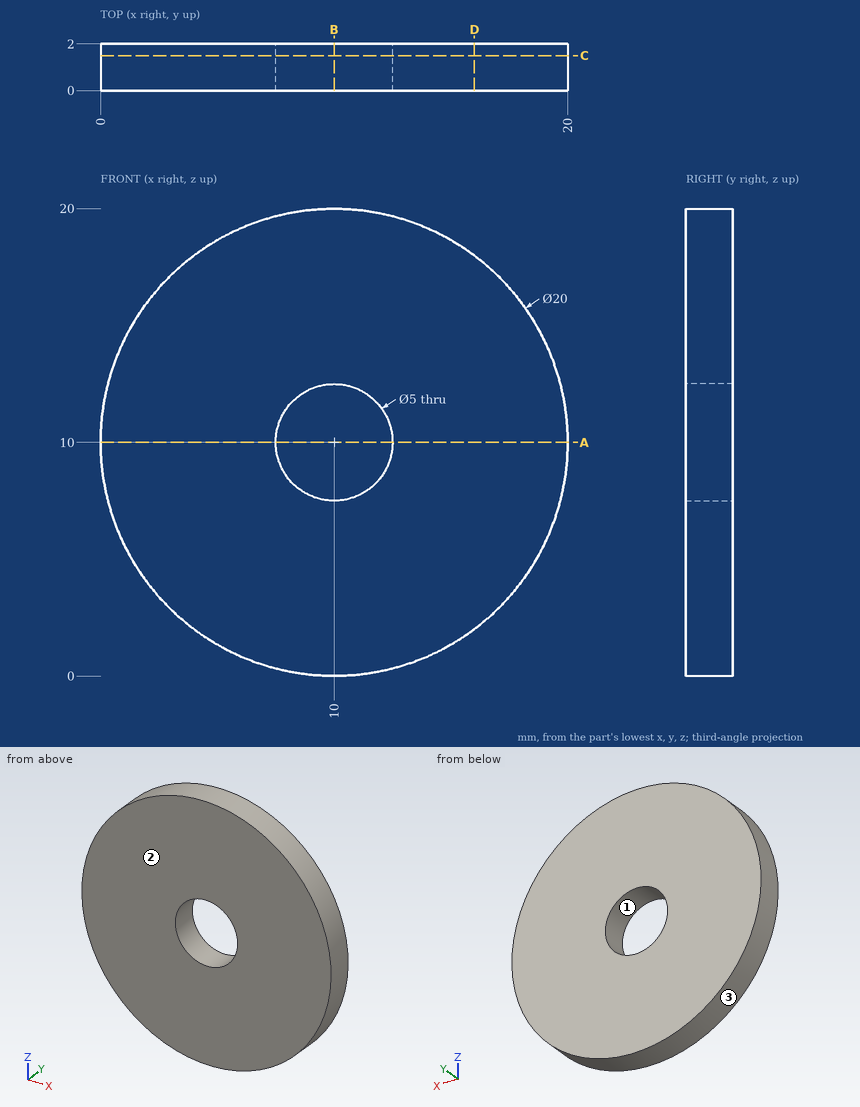
Can you work these out from the drawing? Everything is in mm from the part's minimum corner. Give positions to 0.01 mm unless a question says otherwise; leave off trailing zeros. Order: outer loops, then holes, each group sorted by start corner. A loop starts at its lowest first (then second) coordinate and runs counter-clockwise, first axis right, second up.
1. Will these pins go through, and if not, where does the flat tip stop? P1, Ø1, axis at y = 1.5, z = 17, coming from the +X side; P2, Ø1, axis at x = 6.5, y = 1, coming from the +Z side; P3, Ø1, axis at y = 1.5, z = 3, coming from the -X side; P4, Ø3, axis at x = 10, z = 10, coming from the +Y side (3 decimals).
2. We'd pull the mould along Z, two halves only. Please class the marked faces 1, 2 and 3: pulls with the +Z half, pulls with the -Z half, needs draft (parallel to the pull), parting line crosses it, or undercut.
3. Suppose I cut it at B-B (x = 10). List the corners of the cut face in (y, z) for me, plus the area to 3 significant figures.
4. I need wall thicknesses on L1, parallel to X at y = 0.9, z = 10; L2, parallel to Z at x = 11.75, y = 1; L3, parallel to Z at x = 9, y = 0.7. Which ranges of each line are inside material? Lowest first, please.
5. Suppose I cut it at D-D (x = 16). List the corners of the cut face in (y, z) for me.
6. Suppose I cut it at C-C (y = 1.5). List the corners of the cut face in (x, z) for me, plus the area to 3 significant figures.
7. Suppose I cut it at A-A (z = 10). List the corners of the cut face in (x, y) for me.
Solved:
1. P1: stops at x = 17.6
1. P2: stops at z = 19.54
1. P3: stops at x = 2.4
1. P4: passes through
2. face 1: undercut
2. face 2: needs draft
2. face 3: parting line crosses it
3. outline: (0, 0) - (2, 0) - (2, 7.5) - (0, 7.5) - close; (0, 12.5) - (2, 12.5) - (2, 20) - (0, 20) - close
3. area: 30.0 mm2
4. L1: x = 0 to 7.5, 12.5 to 20
4. L2: z = 0.15 to 8.21, 11.79 to 19.85
4. L3: z = 0.05 to 7.71, 12.29 to 19.95
5. outline: (0, 2) - (2, 2) - (2, 18) - (0, 18) - close
6. outline: circle Ø20 at (10, 10); hole circle Ø5 at (10, 10)
6. area: 295 mm2
7. outline: (0, 0) - (7.5, 0) - (7.5, 2) - (0, 2) - close; (12.5, 0) - (20, 0) - (20, 2) - (12.5, 2) - close
